The model under review builds one solid part; all positions refer to its coordinate system, in mm. A direction names the side the tool comes from. Coordinates: 2 decimals unless noted, no trailing zeros. Write each loop counter-clockwise with the first axis right and the second up, starting at its lowest first coordinate (ties: lowest second). Pieces come first, ordered by that corner, then holes. Notation, with made-up numbers: M 70.5,56.5 L 102.5,56.5 A18 cw 102.5,80.5 Z; hole C -3,31.25 d8. An arc over 180 degrees is marked long. Answer as a JSON object with one key per item and string values.
```python
from build123d import *

# Parameters (mm, degrees)
SKETCH_1_R          = 31
EXTRUDE_2_DEPTH     = 2
SKETCH_2_R          = 32
EXTRUDE_3_DEPTH     = 1
EXTRUDE_START       = 1
SKETCH_3_R          = 32
EXTRUDE_4_DEPTH     = 1
SKETCH_6_R          = 15
EXTRUDE_6_DEPTH     = 6
CUT_EXTRUDE_4_DEPTH = 47.346520905
CUT_EXTRUDE_5_DEPTH = 46.650848842
FILLET_1_R          = 1


with BuildPart() as part:
    # Эскиз1 → Бобышка-Вытянуть2 (new body)
    with BuildSketch(Plane.XY):
        Circle(SKETCH_1_R)
    extrude(amount=EXTRUDE_2_DEPTH)

    # Эскиз2 → Бобышка-Вытянуть3 (add)
    with BuildSketch(Plane.XY.offset(2)):
        Circle(SKETCH_2_R)
    extrude(amount=EXTRUDE_3_DEPTH)

    # Эскиз3 → Бобышка-Вытянуть4 (add)
    with BuildSketch(Plane(origin=(0, 0, 0), x_dir=(-1, 0, 0), z_dir=(0, 0, -1)).offset(EXTRUDE_START)):
        with Locations(Location((0, 0, 0), (0, 0, 180))):
            Circle(SKETCH_3_R)
    extrude(amount=-EXTRUDE_4_DEPTH)

    # Эскиз6 → Бобышка-Вытянуть6 (add)
    with BuildSketch(Plane.XY.offset(3)):
        Circle(SKETCH_6_R)
    extrude(amount=EXTRUDE_6_DEPTH)

    # Эскиз4 → Вырез-Вытянуть4 (cut, through all)
    with BuildSketch(Plane(origin=(0, 0, -1), x_dir=(-1, 0, 0), z_dir=(0, 0, -1))):
        with BuildLine():
            Line((2.437211521, 2.15), (-2.437211521, 2.15))
            ThreePointArc((-2.437211521, 2.15), (0, -3.25), (2.437211521, 2.15))
        make_face()
    extrude(amount=-CUT_EXTRUDE_4_DEPTH, mode=Mode.SUBTRACT)

    # Эскиз7 → Вырез-Вытянуть5 (cut, through all)
    with BuildSketch(Plane.XY.offset(3)):
        with BuildLine():
            Line((-1.196907114, 18.285650075), (4.924848525, 24.115212052))
            ThreePointArc((4.924848525, 24.115212052), (5.321696385, 25.650338094), (4.119277954, 26.683919299))
            ThreePointArc((4.119277954, 26.683919299), (2.505413728, 26.883506134), (0.882461302, 26.985575074))
            ThreePointArc((0.882461302, 26.985575074), (0.120845833, 26.806306653), (-0.446883349, 26.267902657))
            Line((-0.446883349, 26.267902657), (-4.238854139, 20.055785457))
            ThreePointArc((-4.238854139, 20.055785457), (-4.207002942, 18.442797843), (-2.730955491, 17.791623931))
            ThreePointArc((-2.730955491, 17.791623931), (-2.395744761, 17.839854457), (-2.059685964, 17.881769871))
            ThreePointArc((-2.059685964, 17.881769871), (-1.595382366, 18.013397906), (-1.196907114, 18.285650075))
        make_face()
        with BuildLine():
            Line((8.35918988, 18.717007219), (15.078349566, 21.513851098))
            ThreePointArc((15.078349566, 21.513851098), (15.854118052, 21.61572624), (16.575649243, 21.313091099))
            ThreePointArc((16.575649243, 21.313091099), (17.828650719, 20.276568091), (19.016980106, 19.166493358))
            ThreePointArc((19.016980106, 19.166493358), (19.382233263, 17.623544777), (18.158852151, 16.61486304))
            Line((18.158852151, 16.61486304), (9.779717246, 15.496926014))
            ThreePointArc((9.779717246, 15.496926014), (9.297318186, 15.510887259), (8.844319668, 15.677308749))
            ThreePointArc((8.844319668, 15.677308749), (8.547805127, 15.840928871), (8.248264758, 15.99894148))
            ThreePointArc((8.248264758, 15.99894148), (7.436867708, 17.393351165), (8.35918988, 18.717007219))
        make_face()
        with BuildLine():
            Line((17.764307483, 10.228968392), (24.844165441, 8.542239649))
            ThreePointArc((24.844165441, 8.542239649), (25.531656036, 8.168673095), (25.937502559, 7.499730729))
            ThreePointArc((25.937502559, 7.499730729), (26.341949109, 5.924670212), (26.650842222, 4.328118399))
            ThreePointArc((26.650842222, 4.328118399), (26.039415812, 2.865156358), (24.456791453, 2.768201066))
            Line((24.456791453, 2.768201066), (17.020822019, 6.788902937))
            ThreePointArc((17.020822019, 6.788902937), (16.638759195, 7.083744875), (16.370095793, 7.484648537))
            ThreePointArc((16.370095793, 7.484648537), (16.226383986, 7.791306871), (16.076928218, 8.095207168))
            ThreePointArc((16.076928218, 8.095207168), (16.240107663, 9.700235519), (17.764307483, 10.228968392))
        make_face()
        with BuildLine():
            Line((20.384063414, -2.166188691), (25.12035454, -7.692217006))
            ThreePointArc((25.12035454, -7.692217006), (25.456969204, -8.398535529), (25.392111481, -9.178271872))
            ThreePointArc((25.392111481, -9.178271872), (24.79351827, -10.690250315), (24.104988437, -12.16345068))
            ThreePointArc((24.104988437, -12.16345068), (22.750426568, -12.987624407), (21.413067675, -12.135819628))
            Line((21.413067675, -12.135819628), (17.760551297, -4.512250316))
            ThreePointArc((17.760551297, -4.512250316), (17.624759723, -4.049147284), (17.643051725, -3.566893022))
            ThreePointArc((17.643051725, -3.566893022), (17.707035676, -3.234329538), (17.764751533, -2.900621137))
            ThreePointArc((17.764751533, -2.900621137), (18.840178472, -1.698040395), (20.384063414, -2.166188691))
        make_face()
        with BuildLine():
            Line((15.21779995, -13.733935321), (15.801422014, -20.988508213))
            ThreePointArc((15.801422014, -20.988508213), (15.658585386, -21.757789037), (15.147796863, -22.350486576))
            ThreePointArc((15.147796863, -22.350486576), (13.774806152, -23.221858571), (12.351848368, -24.00899502))
            ThreePointArc((12.351848368, -24.00899502), (10.771547634, -23.879574082), (10.190279849, -22.404369706))
            Line((10.190279849, -22.404369706), (11.716353639, -14.089877314))
            ThreePointArc((11.716353639, -14.089877314), (11.87870108, -13.635402806), (12.176961563, -13.256002682))
            ThreePointArc((12.176961563, -13.256002682), (12.424201579, -13.024561994), (12.667043564, -12.788510755))
            ThreePointArc((12.667043564, -12.788510755), (14.243941459, -12.447722593), (15.21779995, -13.733935321))
        make_face()
        with BuildLine():
            Line((4.238854139, -20.055785457), (0.446883349, -26.267902657))
            ThreePointArc((0.446883349, -26.267902657), (-0.120845833, -26.806306653), (-0.882461302, -26.985575074))
            ThreePointArc((-0.882461302, -26.985575074), (-2.505413728, -26.883506134), (-4.119277954, -26.683919299))
            ThreePointArc((-4.119277954, -26.683919299), (-5.321696385, -25.650338094), (-4.924848525, -24.115212052))
            Line((-4.924848525, -24.115212052), (1.196907114, -18.285650075))
            ThreePointArc((1.196907114, -18.285650075), (1.595382366, -18.013397906), (2.059685964, -17.881769871))
            ThreePointArc((2.059685964, -17.881769871), (2.395744761, -17.839854457), (2.730955491, -17.791623931))
            ThreePointArc((2.730955491, -17.791623931), (4.207002942, -18.442797843), (4.238854139, -20.055785457))
        make_face()
        with BuildLine():
            Line((-8.35918988, -18.717007219), (-15.078349566, -21.513851098))
            ThreePointArc((-15.078349566, -21.513851098), (-15.854118052, -21.61572624), (-16.575649243, -21.313091099))
            ThreePointArc((-16.575649243, -21.313091099), (-17.828650719, -20.276568091), (-19.016980106, -19.166493358))
            ThreePointArc((-19.016980106, -19.166493358), (-19.382233263, -17.623544777), (-18.158852151, -16.61486304))
            Line((-18.158852151, -16.61486304), (-9.779717246, -15.496926014))
            ThreePointArc((-9.779717246, -15.496926014), (-9.297318186, -15.510887259), (-8.844319668, -15.677308749))
            ThreePointArc((-8.844319668, -15.677308749), (-8.547805127, -15.840928871), (-8.248264758, -15.99894148))
            ThreePointArc((-8.248264758, -15.99894148), (-7.436867708, -17.393351165), (-8.35918988, -18.717007219))
        make_face()
        with BuildLine():
            Line((-17.764307483, -10.228968392), (-24.844165441, -8.542239649))
            ThreePointArc((-24.844165441, -8.542239649), (-25.531656036, -8.168673095), (-25.937502559, -7.499730729))
            ThreePointArc((-25.937502559, -7.499730729), (-26.341949109, -5.924670212), (-26.650842222, -4.328118399))
            ThreePointArc((-26.650842222, -4.328118399), (-26.039415812, -2.865156358), (-24.456791453, -2.768201066))
            Line((-24.456791453, -2.768201066), (-17.020822019, -6.788902937))
            ThreePointArc((-17.020822019, -6.788902937), (-16.638759195, -7.083744875), (-16.370095793, -7.484648537))
            ThreePointArc((-16.370095793, -7.484648537), (-16.226383986, -7.791306871), (-16.076928218, -8.095207168))
            ThreePointArc((-16.076928218, -8.095207168), (-16.240107663, -9.700235519), (-17.764307483, -10.228968392))
        make_face()
        with BuildLine():
            Line((-20.384063414, 2.166188691), (-25.12035454, 7.692217006))
            ThreePointArc((-25.12035454, 7.692217006), (-25.456969204, 8.398535529), (-25.392111481, 9.178271872))
            ThreePointArc((-25.392111481, 9.178271872), (-24.79351827, 10.690250315), (-24.104988437, 12.16345068))
            ThreePointArc((-24.104988437, 12.16345068), (-22.750426568, 12.987624407), (-21.413067675, 12.135819628))
            Line((-21.413067675, 12.135819628), (-17.760551297, 4.512250316))
            ThreePointArc((-17.760551297, 4.512250316), (-17.624759723, 4.049147284), (-17.643051725, 3.566893022))
            ThreePointArc((-17.643051725, 3.566893022), (-17.707035676, 3.234329538), (-17.764751533, 2.900621137))
            ThreePointArc((-17.764751533, 2.900621137), (-18.840178472, 1.698040395), (-20.384063414, 2.166188691))
        make_face()
        with BuildLine():
            Line((-15.21779995, 13.733935321), (-15.801422014, 20.988508213))
            ThreePointArc((-15.801422014, 20.988508213), (-15.658585386, 21.757789037), (-15.147796863, 22.350486576))
            ThreePointArc((-15.147796863, 22.350486576), (-13.774806152, 23.221858571), (-12.351848368, 24.00899502))
            ThreePointArc((-12.351848368, 24.00899502), (-10.771547634, 23.879574082), (-10.190279849, 22.404369706))
            Line((-10.190279849, 22.404369706), (-11.716353639, 14.089877314))
            ThreePointArc((-11.716353639, 14.089877314), (-11.87870108, 13.635402806), (-12.176961563, 13.256002682))
            ThreePointArc((-12.176961563, 13.256002682), (-12.424201579, 13.024561994), (-12.667043564, 12.788510755))
            ThreePointArc((-12.667043564, 12.788510755), (-14.243941459, 12.447722593), (-15.21779995, 13.733935321))
        make_face()
    extrude(amount=-CUT_EXTRUDE_5_DEPTH, mode=Mode.SUBTRACT)

    # Скругление1
    fillet_1_edges = [part.edges().sort_by_distance(p)[0] for p in [
        (-15, 0, 9),
    ]]
    fillet(fillet_1_edges, radius=FILLET_1_R)


solid = part.part
```
(1) Add section B-B on z = 5.25. Give the boundary of the cut face in (x, y).
Results list:
{"outline": "C 0,0 d30; hole M -2.44,2.15 A3.25 ccw long 2.44,2.15 Z"}
(2) Add section A-A on y = 0. Give the boundary of the cut face in (x, z).
Results list:
{"outline": "M -32,-1 L -3.25,-1 L -3.25,9 L -14,9 A1 ccw -15,8 L -15,3 L -32,3 L -32,2 L -31,2 L -31,0 L -32,0 Z; M 3.25,-1 L 32,-1 L 32,0 L 31,0 L 31,2 L 32,2 L 32,3 L 15,3 L 15,8 A1 ccw 14,9 L 3.25,9 Z"}
(3) For faces 1 (the face through (2.53, 26.88, 1.03)), 2 (the face through (7, 0, -1)), list the 3-axis set-ups (+Z, -Z, +X, -X, +Y, -Y) from which the entire face can be reached by the end or side of a thin tool; tool diameter is ignored.
Results list:
{"face 1": "+Z, -Z", "face 2": "-Z, +X, -X, +Y, -Y"}
(4) For pin 1 Ø3 at (x, z) = (-10, 7.5) entering from +Y; pin 2 Ø2 at (y, z) = (11.5, 5.5) entering from +X; pin 3 Ø1.5 at (y, z) = (11, 4) entering from -X, all flat-tipped, find the tip position at first contact; note any pin that passes through.
Results list:
{"pin 1": "y = 12.36", "pin 2": "x = 10.71", "pin 3": "x = -10.95"}
(5) Draft analysis for pull direction Y (two halves, no side actions). For faces 3 (the face through (-4.036, 30.736, 0.986)), 4 (the face through (14, -7, 3)), 5 (the face through (19.39, 17.65, 1.03)), state which applies: released by +Y, released by -Y, zero draft, split by the parting line, or undercut.
Results list:
{"face 3": "split by the parting line", "face 4": "zero draft", "face 5": "undercut"}
(6) Wall thickness on line 1 along Y through (x, z) = (19.5, 1); line 2 along X through (y, z) = (8, 2.25); line 3 along Y through (x, z) = (0, 5.25): over which ranges is each line inside the solid? List them lowest first. Write a range as from..to.
Results list:
{"line 1": "-24.1..-8.14, -1.66..5.45, 9.82..24.1", "line 2": "-30.98..-25.32, -19.43..16.12, 25.68..30.98", "line 3": "-15..-3.25, 2.15..15"}
(7) Add section C-C on z = 1.25. Count the separate pieces of the cut face and the enclosed holes in it, and give its area (3 significant figures).
Results list:
{"separate pieces": "1", "enclosed holes": "11", "area": "2,510 mm²"}
